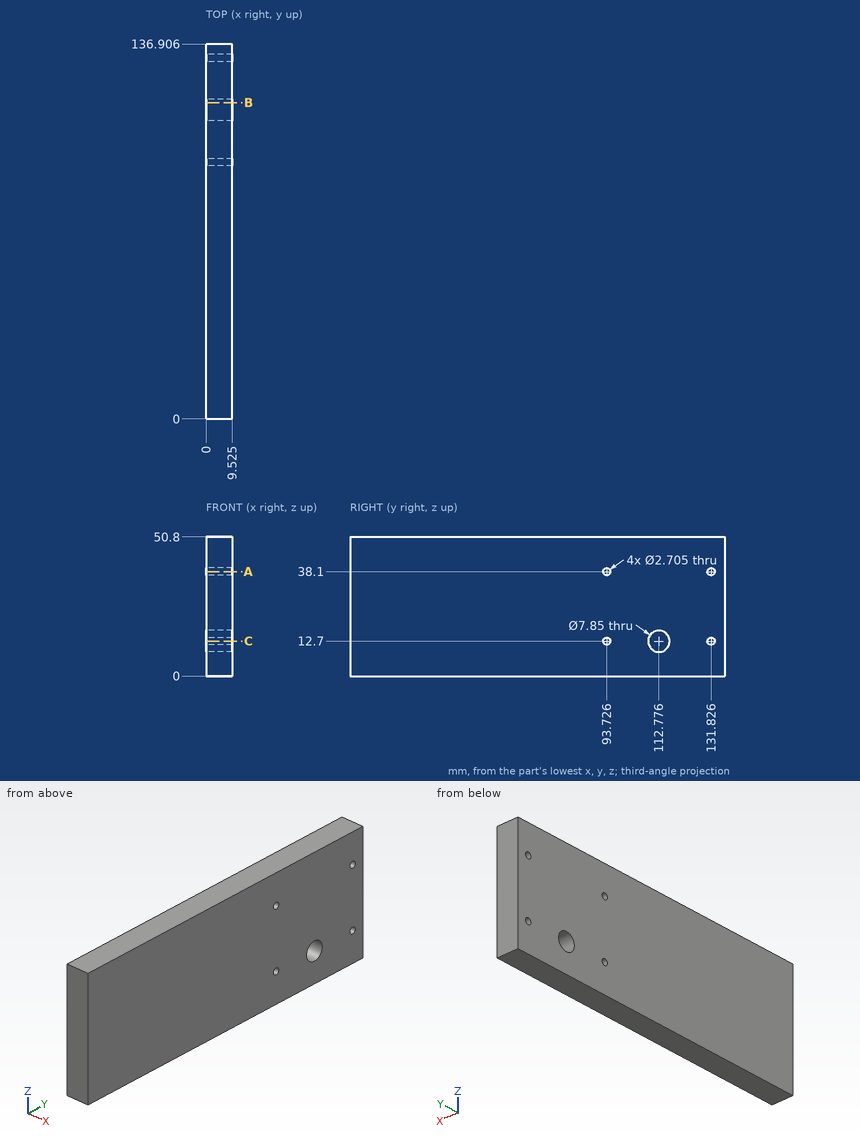
Design review of the part shown in the three views and the two pictorial views. Dimensions are in mm from the part's minimum x, y and z. Coordinates: 2 decimals unless noted, no trailing zeros. Loops run counter-clockwise (first coordinate to the right, second up) from the corner with the lowest first, then second, coordinate; pieces in that order, holes last. Notation, with made-up numbers: (3.5, 84) - (31.5, 84) arc R15 ccw to (31.5, 113) - close; hole circle Ø1 at (38, 76.5). An arc over 180 degrees is marked (long way). Use a Markdown table: item, result. Add a question column.
Item 1: For line 1 (Y direction, x = 5.75, z = 12.7); line 2 (Y direction, x = 6.5, z = 38.1); line 3 (Y direction, x = 1.5, z = 37.5), list the stretches that pass through material, from the lowest coordinate up.
Item 2: We need section A-A (z = 38.1). Give the boundary of the cut face in (x, y) (1 decimal).
Item 3: Insertion check: pin 1 Ø2.5 at (y, z) = (93.726, 38.1) entering from +X. The pin has a flat end and moves straight along its axis. Give the tip position at first contact, or say it passes through.
Item 4: We need section B-B (y = 115.5). Give the boundary of the cut face in (x, z) (3 decimals), and give its area (3 significant figures).
Item 5: We need section C-C (z = 12.7). Give the boundary of the cut face in (x, y) (1 decimal), and give its area (3 significant figures).
Results list:
| question | item | result |
|---|---|---|
| 1 | line 1 | y = 0 to 92.37, 95.08 to 108.85, 116.7 to 130.47, 133.18 to 136.91 |
| 1 | line 2 | y = 0 to 92.37, 95.08 to 130.47, 133.18 to 136.91 |
| 1 | line 3 | y = 0 to 92.51, 94.94 to 130.61, 133.04 to 136.91 |
| 2 | outline | (0, 0) - (9.5, 0) - (9.5, 92.4) - (0, 92.4) - close; (0, 95.1) - (9.5, 95.1) - (9.5, 130.5) - (0, 130.5) - close; (0, 133.2) - (9.5, 133.2) - (9.5, 136.9) - (0, 136.9) - close |
| 3 | pin 1 | passes through |
| 4 | outline | (0, 0) - (9.525, 0) - (9.525, 9.874) - (0, 9.874) - close; (0, 15.526) - (9.525, 15.526) - (9.525, 50.8) - (0, 50.8) - close |
| 4 | area | 430 mm^2 |
| 5 | outline | (0, 0) - (9.5, 0) - (9.5, 92.4) - (0, 92.4) - close; (0, 95.1) - (9.5, 95.1) - (9.5, 108.9) - (0, 108.9) - close; (0, 116.7) - (9.5, 116.7) - (9.5, 130.5) - (0, 130.5) - close; (0, 133.2) - (9.5, 133.2) - (9.5, 136.9) - (0, 136.9) - close |
| 5 | area | 1,180 mm^2 |
